Build history of the part. All positions in model axes, mm. A direction names the side the tool comes from. Give positions to 0.01 mm unless a question says otherwise; leave off trailing zeros. Loops run counter-clockwise (first coordinate to the right, second up) from the corner with the lowest first, then second, coordinate; pieces in that order, holes last. Notation, with made-up numbers: M 53,83.5 L 88,83.5 A28 cw 88,105.5 Z; hole C -14,-25 d8. An arc over 180 degrees is marked long. Put each result on its own line as item: value.
```python
from build123d import *

# Parameters (mm, degrees)
ESQUISSE1_W             = 19
ESQUISSE1_H             = 70
ESQUISSE1_R             = 1.7
BOSS_EXTRU_1_DEPTH      = 2
ESQUISSE2_W             = 65
ESQUISSE2_H             = 60
BOSS_EXTRU_2_DEPTH      = 2
ESQUISSE3_R             = 1.7
ESQUISSE3_R_2           = 1
ENL_V_MAT_EXTRU_1_DEPTH = 2
ESQUISSE4_R             = 1.7
ENL_V_MAT_EXTRU_2_DEPTH = 2
ESQUISSE5_W             = 31.414941094
ESQUISSE5_H             = 20
ENL_V_MAT_EXTRU_3_DEPTH = 10
BOSS_EXTRU_7_DEPTH      = 28
ENL_V_MAT_EXTRU_4_DEPTH = 60
ENL_V_MAT_EXTRU_5_DEPTH = 72
ENL_V_MAT_EXTRU_6_DEPTH = 67
ENL_V_MAT_EXTRU_7_DEPTH = 35
BOSS_EXTRU_11_DEPTH     = 2
ESQUISSE15_R            = 1.7
ENL_V_MAT_EXTRU_8_DEPTH = 10


with BuildPart() as part:
    # Esquisse1 → Boss.-Extru.1 (new body)
    with BuildSketch(Plane.XY):
        with Locations((-2.5, -24.85)):
            Rectangle(ESQUISSE1_W, ESQUISSE1_H)
        Circle(ESQUISSE1_R, mode=Mode.SUBTRACT)
        with Locations((0, -49.7)):
            Circle(ESQUISSE1_R, mode=Mode.SUBTRACT)
    extrude(amount=BOSS_EXTRU_1_DEPTH)

    # Esquisse2 → Boss.-Extru.2 (add)
    with BuildSketch(Plane(origin=(0, 0, 0), x_dir=(-1, 0, 0), z_dir=(0, 0, -1))):
        with Locations((42.768488136, -24.85)):
            Rectangle(ESQUISSE2_W, ESQUISSE2_H)
    extrude(amount=-BOSS_EXTRU_2_DEPTH)

    # Esquisse3 → Enlèv. mat.-Extru.1 (cut)
    with BuildSketch(Plane(origin=(0, 0, 0), x_dir=(-1, 0, 0), z_dir=(0, 0, -1))):
        with Locations((56.248017163, -52.23632124)):
            Circle(ESQUISSE3_R)
        with Locations((25.480085092, -25.094879292)):
            Circle(ESQUISSE3_R_2)
        with Locations((62.780085092, -25.094879292)):
            Circle(ESQUISSE3_R_2)
        with Locations((71.248017163, -52.23632124)):
            Circle(ESQUISSE3_R)
        with Locations((21.945704193, 2.053157955)):
            Circle(ESQUISSE3_R)
        with Locations((26.445704193, 2.053157955)):
            Circle(ESQUISSE3_R)
        with Locations((30.945704193, 2.053157955)):
            Circle(ESQUISSE3_R)
        with Locations((35.445704193, 2.053157955)):
            Circle(ESQUISSE3_R)
        with Locations((72.562852247, -43.246842045)):
            Circle(ESQUISSE3_R)
        with Locations((72.562852247, -22.946842045)):
            Circle(ESQUISSE3_R)
        with Locations((72.562852247, -12.146842045)):
            Circle(ESQUISSE3_R)
        with Locations((72.562852247, 2.053157955)):
            Circle(ESQUISSE3_R)
        with Locations((25.480085092, -52.23632124)):
            Circle(ESQUISSE3_R)
        with Locations((44.580085092, -52.23632124)):
            Circle(ESQUISSE3_R)
        with Locations((39.945704193, 2.053157955)):
            Circle(ESQUISSE3_R)
        with Locations((44.445704193, 2.053157955)):
            Circle(ESQUISSE3_R)
        with Locations((48.945704193, 2.053157955)):
            Circle(ESQUISSE3_R)
        with Locations((53.445704193, 2.053157955)):
            Circle(ESQUISSE3_R)
        with Locations((57.945704193, 2.053157955)):
            Circle(ESQUISSE3_R)
        with Locations((62.445704193, 2.053157955)):
            Circle(ESQUISSE3_R)
        with Locations((66.945704193, 2.053157955)):
            Circle(ESQUISSE3_R)
    extrude(amount=-ENL_V_MAT_EXTRU_1_DEPTH, mode=Mode.SUBTRACT)

    # Esquisse4 → Enlèv. mat.-Extru.2 (cut)
    with BuildSketch(Plane(origin=(0, 0, 0), x_dir=(-1, 0, 0), z_dir=(0, 0, -1))):
        with Locations((16, -49.7)):
            Circle(ESQUISSE4_R)
        with Locations((16, 0)):
            Circle(ESQUISSE4_R)
    extrude(amount=-ENL_V_MAT_EXTRU_2_DEPTH, mode=Mode.SUBTRACT)

    # Esquisse5 → Enlèv. mat.-Extru.3 (cut)
    with BuildSketch(Plane(origin=(0, 0, 0), x_dir=(-1, 0, 0), z_dir=(0, 0, -1))):
        with Locations((44.561017589, -24.85)):
            Rectangle(ESQUISSE5_W, ESQUISSE5_H)
    extrude(amount=-ENL_V_MAT_EXTRU_3_DEPTH, mode=Mode.SUBTRACT)

    # Esquisse9 → Boss.-Extru.7 (add)
    with BuildSketch(Plane.XY.offset(2)):
        Polygon((-3.5, -53.689758583), (-3.5, 3.5), (-28.853547042, 3.5), (-60.346670852, 3.5), (-60.346670852, -53.689758583), (-28.853547042, -53.689758583), align=None)
    extrude(amount=BOSS_EXTRU_7_DEPTH)

    # Esquisse10 → Enlèv. mat.-Extru.4 (cut)
    with BuildSketch(Plane(origin=(0, 3.5, 0), x_dir=(1, 0, 0), z_dir=(0, 1, 0))):
        Polygon((-18.30138002, -2), (-3.5, -2), (-3.5, -23.208493493), align=None)
        Polygon((-8.472856096, -30), (-18.30138002, -9.274207286), (-57.123898362, -2), (-60.855534618, -2), (-60.855534618, -30), (-28.853547042, -30), align=None)
    extrude(amount=-ENL_V_MAT_EXTRU_4_DEPTH, mode=Mode.SUBTRACT)

    # Esquisse11 → Enlèv. mat.-Extru.5 (cut)
    with BuildSketch(Plane(origin=(7, 0, 0), x_dir=(0, 0, -1), z_dir=(1, 0, 0))):
        Polygon((-23.208493493, 3.5), (-2, -5.465834256), (-2, 3.5), align=None)
        Polygon((-2, -44.723924327), (-2, -53.689758583), (-23.208493493, -53.689758583), align=None)
    extrude(amount=-ENL_V_MAT_EXTRU_5_DEPTH, mode=Mode.SUBTRACT)

    # Esquisse12 → Enlèv. mat.-Extru.6 (cut)
    with BuildSketch(Plane(origin=(7, 0, 0), x_dir=(0, 0, -1), z_dir=(1, 0, 0))):
        with BuildLine():
            Line((-2, -15.094879292), (-2, -35.094879292))
            ThreePointArc((-2, -35.094879292), (-6.168544771, -34.184611658), (-9.578191265, -31.619526191))
            Line((-9.578191265, -31.619526191), (-19.578951758, -25.094879292))
            Line((-19.578951758, -25.094879292), (-9.578191265, -18.570232393))
            ThreePointArc((-9.578191265, -18.570232393), (-6.168544771, -16.005146925), (-2, -15.094879292))
        make_face()
    extrude(amount=-ENL_V_MAT_EXTRU_6_DEPTH, mode=Mode.SUBTRACT)

    # Esquisse13 → Enlèv. mat.-Extru.7 (cut)
    with BuildSketch(Plane.XY.offset(2)):
        with BuildLine():
            Line((-60.268488136, -14.85), (-22.770000782, -14.85))
            Line((-22.770000782, -14.85), (-22.770000782, -20.893041237))
            ThreePointArc((-22.770000782, -20.893041237), (-20.480085092, -25.094879292), (-22.770000782, -29.296717346))
            Line((-22.770000782, -29.296717346), (-22.770000782, -34.85))
            Line((-22.770000782, -34.85), (-60.268488136, -34.85))
            Line((-60.268488136, -34.85), (-60.268488136, -14.85))
        make_face()
    extrude(amount=ENL_V_MAT_EXTRU_7_DEPTH, mode=Mode.SUBTRACT)

    # Esquisse14 → Boss.-Extru.11 (add)
    with BuildSketch(Plane(origin=(-13.245694898, 0, 9.244153239), x_dir=(-0.572305295, 0, -0.820040639), z_dir=(0.820040639, 0, -0.572305295))):
        Polygon((8.833895415, -35.094879292), (10.168090758, -35.094879292), (10.168090758, -15.094879292), (8.833895415, -15.094879292), (-13.439734278, -15.094879292), (-13.439734278, -35.094879292), align=None)
    extrude(amount=-BOSS_EXTRU_11_DEPTH)

    # Esquisse15 → Enlèv. mat.-Extru.8 (cut)
    with BuildSketch(Plane(origin=(0, 0, 0), x_dir=(-1, 0, 0), z_dir=(0, 0, -1))):
        with Locations((20.233733499, -50.143649221)):
            Circle(ESQUISSE15_R)
        with Locations((21.376751472, -1.943649221)):
            Circle(ESQUISSE15_R)
        with Locations((72.616751472, -17.553649221)):
            Circle(ESQUISSE15_R)
    extrude(amount=-ENL_V_MAT_EXTRU_8_DEPTH, mode=Mode.SUBTRACT)


solid = part.part
```
Q1. Drop flat-ended pins along their axis: pin 1 Ø0.6 at (y, z) = (-57.5, 1) entering from -X; pin 2 Ø4 at (x, y) = (-17.5, -21.5) entering from +Z; pin 3 Ø4.5 at (x, y) = (-72.62, -17.55) entering from +Z. Give the stop position or say it passes through.
Here are the results:
pin 1: x = -12
pin 2: z = 15.18
pin 3: z = 2
Q2. Tool access for faces 1 (the flat face through (-37.44, -39.77, 5.69)), 2 (the flat face through (-44, -34.85, 1)), 3 (the flat face through (-3, -59.85, 1)), 4 (the cylindrical face through (-16.914, -48.267, 0.986)), 5 (the flat face through (-15.86, -24.95, 8.99)): list every direction of +Z, -Z, +X, -X, +Y, -Y with a clear straight run to the whole face (end or side of a thin tool).
Here are the results:
face 1: +Z, -X, +Y, -Y
face 2: +Z, -Z
face 3: +Z, -Z, +X, -X, -Y
face 4: -Z
face 5: -X
Q3. Slice it at A-A (x = 0). List the corners of the cut face in (y, z).
Here are the results:
outline: M -59.85,0 L -51.4,0 L -51.4,2 L -59.85,2 Z; M -48,0 L -1.7,0 L -1.7,2 L -48,2 Z; M 1.7,0 L 10.15,0 L 10.15,2 L 1.7,2 Z
Q4. Slice it at D-D (x = -53.5). List the corners of the cut face in (y, z).
Here are the results:
outline: M -54.85,0 L -34.85,0 L -34.85,2 L -35.09,2 A10 cw -35.07,2.68 L -45.01,2.68 L -44.72,2 L -54.85,2 Z; M -14.85,0 L 0.35,0 L 0.35,2 L -5.47,2 L -5.18,2.68 L -14.85,2.68 Z; M 3.75,0 L 5.15,0 L 5.15,2 L 3.75,2 Z
Q5. Slice it at B-B (y = -30). List the corners of the cut face in (x, z), and give its area (3 significant figures).
Here are the results:
outline: M -75.27,0 L -60.27,0 L -60.27,2 L -75.27,2 Z; M -28.85,0 L 7,0 L 7,2 L -18.3,2 L -3.5,23.21 L -3.5,30 L -8.47,30 L -16.98,12.06 L -13.72,12.06 L -20.71,2.05 L -20.63,2 L -28.85,2 Z
area: 248 mm²
Q6. Slice it at C-C (z = 13.5). List the corners of the cut face in (x, y).
Here are the results:
outline: M -16.3,-49.59 L -10.28,-49.59 L -10.28,-0.6 L -16.3,-0.6 L -16.3,-21.13 L -12.71,-21.13 L -12.71,-29.06 L -16.3,-29.06 Z
Q7. Probe line 1 (Y direction, x = 0, z = 1.2); line 2 (Z direction, x = -68, y = -15); line 3 (Z direction, x = -11, y = -41). List the from-to ranges inside material, lowest first. Write a range as from..to.
Here are the results:
line 1: -59.85..-51.4, -48..-1.7, 1.7..10.15
line 2: 0..2
line 3: 0..2, 12.46..24.67
Q8. Mould opens along Y. For faces 6 (the flat face through (-75.268, -25, 1)), 7 (the cylindrical face through (-26.39, -50.8, 0.99)), 8 (the flat face through (-24.229, -47.235, 7.941)) say: pulls with the +Y half, pulls with the -Y half, needs draft (parallel to the pull), parting line crosses it, or undercut.
Here are the results:
face 6: needs draft
face 7: undercut
face 8: pulls with the -Y half
